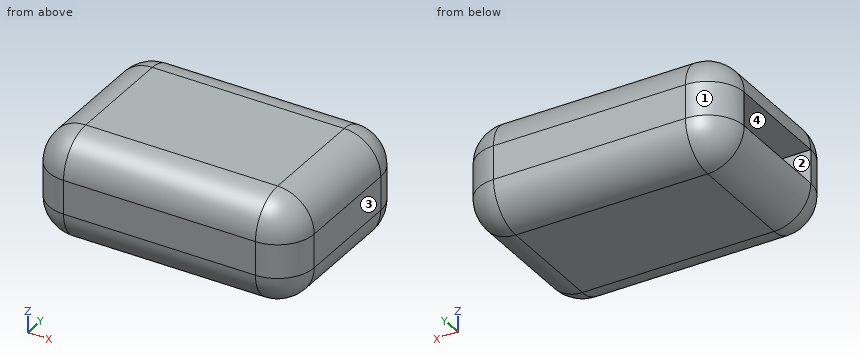
from build123d import *

# Parameters (mm, degrees)
F0_W     = 36.83
F0_H     = 25.4
F1_DEPTH = 14.859
F2_W     = 15.24
F2_H     = 4.699
F3_DEPTH = 18.542
F4_DEPTH = 16.256
F5_R     = 5.07999


# Not quite as in the source:
# - a fillet or chamfer is up to 0.001 mm smaller than in the source, because OpenCascade refuses the exact size


with BuildPart() as f1:
    # F0 (on Top) → F1 (new body)
    with BuildSketch(Plane.XY):
        Rectangle(F0_W, F0_H)
    extrude(amount=F1_DEPTH)

    # F2 (on Right) → F3 (cut)
    with BuildSketch(Plane.YZ):
        with Locations((0, 7.4295)):
            Rectangle(F2_W, F2_H)
    extrude(amount=-F3_DEPTH, mode=Mode.SUBTRACT)

    # F2 (on Right) → F4 (cut)
    with BuildSketch(Plane.YZ):
        with Locations((0, 7.4295)):
            Rectangle(F2_W, F2_H)
    extrude(amount=F4_DEPTH, mode=Mode.SUBTRACT)

    # F5 (radius 5.08 in the source; OpenCascade refuses exactly that, so slightly less here)
    f5_edges = [f1.edges().sort_by_distance(p)[0] for p in [
        (0, -12.7, 14.859),
        (18.415, 0, 14.859),
        (18.415, -12.7, 7.4295),
        (18.415, 0, 0),
        (18.415, 12.7, 7.4295),
        (0, 12.7, 0),
        (0, -12.7, 0),
        (0, 12.7, 14.859),
        (-18.415, 0, 14.859),
        (-18.415, 12.7, 7.4295),
        (-18.415, 0, 0),
        (-18.415, -12.7, 7.4295),
    ]]
    fillet(f5_edges, radius=F5_R)


solid = f1.part
Could you check a few things on this model? Use its own coordinates, in mm. Face numbers are marked on the shaded views. Give positions to 0.01 mm unless a question says otherwise; leave off trailing zeros. Order: outer loops, then holes, each group sorted by start corner. A loop starts at its lowest first (then second) coordinate and runs counter-clockwise, first axis right, second up.
Item 1: If we section it at D-D, the plane y = 9: Write out the boundary of the cut face in (x, z) (3 decimals), plus the area to 3 significant figures.
Item 2: If we section it at A-A, the plane x = 1: Write out the boundary of the cut face in (y, z), plus the area to 3 significant figures.
Item 3: I need wall thicknesses on line 1 (Y direction, x = -9, z = 6); line 2 (Z direction, x = 7, y = 3.5); line 3 (X direction, y = 5, z = 9.25) (3 decimals). Which ranges of each line are inside material? Lowest first, please.
Item 4: I'm going to push flat-ended pins straight in: pin 1 (2.5 mm diameter, centred on y = 1, z = 6.5, fed in from -X); pin 2 (5 mm diameter, centred on y = 2, z = 13.5, fed in from -X). Where does each tip first touch, or does it pass through?
Item 5: If we mould it in two halves opening along Y, with no side actions, what happens to the marked faces 1, 2, 3 and 4? For each: pulls with the +Y half, pulls with the -Y half, needs draft (parallel to the pull), parting line crosses it, or undercut.
Values:
1. outline: (-18.224, 5.08) arc R4.889 ccw to (-13.335, 0.191) - (13.335, 0.191) arc R4.889 ccw to (18.224, 5.08) - (18.224, 9.779) arc R4.889 ccw to (13.335, 14.668) - (-13.335, 14.668) arc R4.889 ccw to (-18.224, 9.779) - close
1. area: 507 mm2
2. outline: (-12.7, 5.08) arc R5.08 ccw to (-7.62, 0) - (7.62, 0) arc R5.08 ccw to (12.7, 5.08) - (12.7, 9.78) arc R5.08 ccw to (7.62, 14.86) - (-7.62, 14.86) arc R5.08 ccw to (-12.7, 9.78) - close; hole (-7.62, 5.08) - (7.62, 5.08) - (7.62, 9.78) - (-7.62, 9.78) - close
2. area: 284 mm2
3. line 1: y = -12.7 to -7.62, 7.62 to 12.7
3. line 2: z = 0 to 5.08, 9.78 to 14.86
3. line 3: x = 16.256 to 18.415
4. pin 1: stops at x = 16.26
4. pin 2: stops at x = -18.27
5. face 1: pulls with the +Y half
5. face 2: undercut
5. face 3: needs draft
5. face 4: undercut
